from build123d import *

# Parameters (mm, degrees)
CHAMFER1_SIZE = 1
SCALE1_SCALE  = 0.828947368


with BuildPart() as part:
    # Sketch1 → Revolve1 (revolve)
    with BuildSketch(Plane.XY, mode=Mode.PRIVATE) as revolve1_sk:
        Polygon((-41.050847458, 26.110169492), (-8.050847458, 26.110169492), (-8.050847458, 20.110169492), (-41.050847458, 20.110169492), (-48.050847458, 20.110169492), (-48.050847458, 27.110169492), (-41.050847458, 27.110169492), align=None)
    revolve(revolve1_sk.sketch.rotate(Axis((-48.881355932, 20.110169492, 0), (1, 0, 0)), 90), axis=Axis((-48.881355932, 20.110169492, 0), (1, 0, 0)))

    # Chamfer1
    chamfer1_edges = [part.edges().sort_by_distance(p)[0] for p in [
        (-8.050847458, 20.110169492, -6),
    ]]
    chamfer(chamfer1_edges, length=CHAMFER1_SIZE)


with BuildPart() as part_1:
    # Scale1: scaled about (-29.108266601, 20.110169492, 0)
    add(part.part.scale(SCALE1_SCALE).moved(Location((-4.979045615, 3.439897422, 0))))


solid = part_1.part
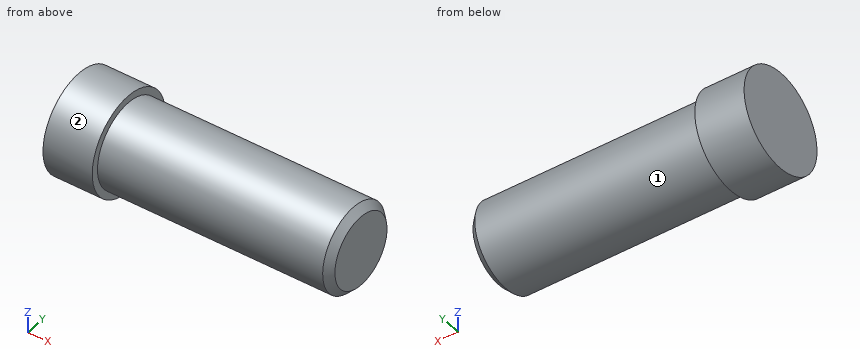
Read the model definition and answer for the solid it produces. Units are mm, in the model's axes. Face numbers are marked on the shaded views. A direction names the side the tool comes from. Give positions to 0.01 mm unless a question says otherwise; leave off trailing zeros. Write each loop counter-clockwise with the first axis right and the second up, starting at its lowest first coordinate (ties: lowest second). Pieces come first, ordered by that corner, then holes. Notation, with made-up numbers: (66.25, -11.75) -> (120.25, -11.75) arc R25 ccw to (120.25, 4.25) -> close; hole circle Ø10 at (3.25, 23). An arc over 180 degrees is marked (long way). Answer as a JSON object with one key per item and string values. Group by question number.
1) Find section A-A (z = 0). Write down the section's boundary in (x, y).
2) Consider L1, parallel to X at y = 24.25, z = -3.75; L2, parallel to Y at x = -42, z = 3; L3, parallel to X at y = 15.75, z = 2. Determine where each line is inside the solid, lowest interval first. Write a range as from..to.
3) Find section B-B (x = -13.5). Write down the section's boundary in (y, z), and give its area (3 significant figures).
4) A tool of negligible diameter and unlimited length cuts with its end or side. For the marked faces 1 and 2, from which of +Z, -Z, +X, -X, +Y, -Y can it reach the whole face along a straight path? Write none if from no direction.
5) Each of these flat-tipped pins is pushed along its axis until it touches: P1, Ø6, axis at x = -24.5, z = 2, coming from the +Y side; P2, Ø2, axis at x = -37.5, y = 19, coming from the -Z side; P3, Ø1, axis at x = -16, y = 15.5, coming from the -Z side. Where does it stop, or does it pass through?
Values follow:
{
 "1": {"outline": "(-44.81, 14.31) -> (-39.01, 14.31) -> (-39.01, 15.14) -> (-12.48, 15.14) -> (-11.65, 15.97) -> (-11.65, 24.25) -> (-12.48, 25.08) -> (-39.01, 25.08) -> (-39.01, 25.91) -> (-44.81, 25.91) -> close"},
 "2": {"L1": "x = -44.81..-39.01", "L2": "y = 15.14..25.08", "L3": "x = -44.81..-12.31"},
 "3": {"outline": "circle Ø9.95 at (20.11, 0)", "area": "77.7 mm2"},
 "4": {"face 1": "+X", "face 2": "+X, -X"},
 "5": {"P1": "stops at y = 25.08", "P2": "stops at z = -4.97", "P3": "stops at z = -2.8"}
}
